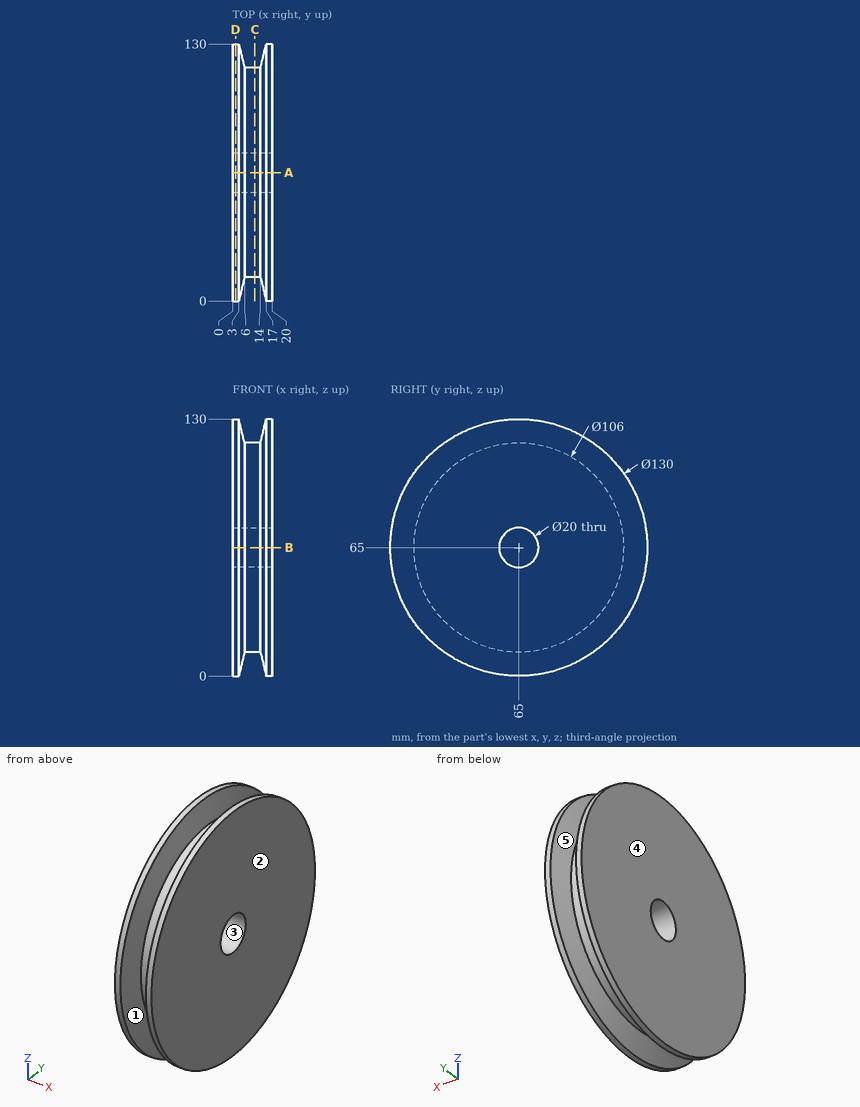
Input: dimensioned drawing with shaded views. Units: mm. Origin: part minimum x, y, z. A direction names the side the tool comes from. Coordinates: 2 decimals unless noted, no trailing zeros. Write each loop counter-clockwise with the first axis right and the second up, starting at its lowest first coordinate (ties: lowest second). Pieces come first, ordered by that corner, then holes. Notation, with made-up numbers: (84.5, 32.25) -> (115.5, 32.25) arc R19 cw to (115.5, 63.25) -> close; hole circle Ø5 at (57.25, -29). An arc over 180 degrees is marked (long way). Return JSON: item names as keys, results as strings. Group by question number.
1) Set-up query: the marked faces 4 and 5. Return all of +Z, -Z, +X, -X, +Y, -Y with unobstructed straight access to the full face (end or side cutting, diameter ignored); none if empty.
2) Section query A-A, the plane y = 65. Return loops of the section in (x, z), plus the area to 3 significant figures.
3) Section query C-C, the plane x = 11.25. Return loops of the section in (y, z), plus the area to 3 significant figures.
4) Contact query for flat-ended pins moving along their axis: P1, Ø12, axis at x = 8, z = 44, coming from the -Y side; P2, Ø2, axis at x = 8, y = 76.5, coming from the +Z side; P3, Ø2, axis at x = 9.5, y = 52.5, coming from the -Z side. Output: stop coordinate, or through.
5) Ray query, line 1 along Y through (x, z) = (8.75, 65); line 2 along X through (y, z) = (92, 113.5); line 3 along Y through (x, z) = (18.5, 74). Return the intervals inside material, ascending.
6) Mould query, pull axis Y, two halves, no side actions, for the marked faces 1, 2 and 3. Classes: +Y half, -Y half, draft (parallel to the pull), parting line (faces both ways), or undercut.
7) Section query D-D, the plane x = 1.5. Return loops of the section in (y, z), plus the area to 3 significant figures.
From the geometry:
{
 "1": {"face 4": "+Z, -Z, -X, +Y, -Y", "face 5": "none"},
 "2": {"outline": "(0, 0) -> (3, 0) -> (6, 12) -> (14, 12) -> (17, 0) -> (20, 0) -> (20, 55) -> (0, 55) -> close; (0, 75) -> (20, 75) -> (20, 130) -> (17, 130) -> (14, 118) -> (6, 118) -> (3, 130) -> (0, 130) -> close", "area": "1,940 mm²"},
 "3": {"outline": "circle Ø106 at (65, 65); hole circle Ø20 at (65, 65)", "area": "8,510 mm²"},
 "4": {"P1": "y = 2.45", "P2": "z = 116.95", "P3": "z = 13.26"},
 "5": {"line 1": "12 to 55, 75 to 118", "line 2": "0 to 5.37, 14.63 to 20", "line 3": "0.63 to 60.64, 69.36 to 129.37"},
 "6": {"face 1": "parting line", "face 2": "draft", "face 3": "undercut"},
 "7": {"outline": "circle Ø130 at (65, 65); hole circle Ø20 at (65, 65)", "area": "13,000 mm²"}
}
